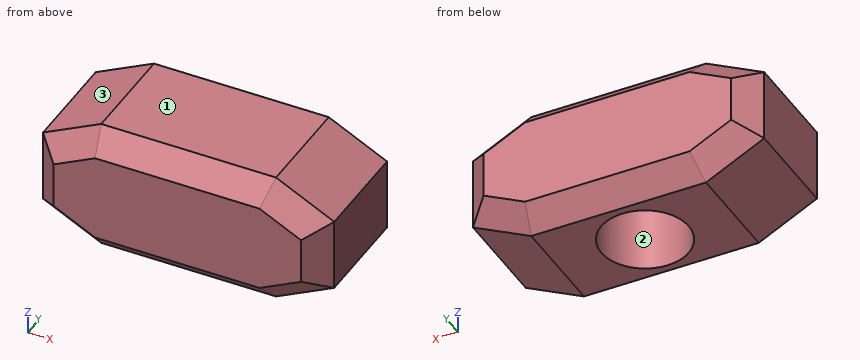
from build123d import *

# Parameters (mm, degrees)
F1_DEPTH = 20
F2_SIZE  = 3
F3_R     = 6
F4_DEPTH = 10
F5_R     = 0.5


with BuildPart() as f1:
    # F0 (on Front) → F1 (new body)
    with BuildSketch(Plane.XZ):
        Polygon((0, 4), (8, 0), (32, 0), (40, 4), (40, 14), (32, 18), (8, 18), (0, 14), align=None)
    extrude(amount=F1_DEPTH)

    # F2
    f2_edges = [f1.edges().sort_by_distance(p)[0] for p in [
        (4, -20, 2),
        (20, -20, 0),
        (36, -20, 2),
        (40, -20, 9),
        (36, -20, 16),
        (20, -20, 18),
        (4, -20, 16),
        (0, -20, 9),
        (4, 0, 2),
        (20, 0, 0),
        (36, 0, 2),
        (40, 0, 9),
        (36, 0, 16),
        (20, 0, 18),
        (4, 0, 16),
        (0, 0, 9),
    ]]
    chamfer(f2_edges, length=F2_SIZE)

    # F3 (on face) → F4 (cut)
    with BuildSketch(Plane(origin=(0, 0, 0), x_dir=(1, 0, 0), z_dir=(0, 0, -1))):
        with Locations((20, 10)):
            Circle(F3_R)
    extrude(amount=-F4_DEPTH, mode=Mode.SUBTRACT)

    # F5
    f5_edges = [f1.edges().sort_by_distance(p)[0] for p in [
        (14, -10, 10),
    ]]
    fillet(f5_edges, radius=F5_R)


solid = f1.part
Work out the finished part from the listing and answer in its coordinate system (mm). Face numbers are marked on the shaded views. Give positions to 0.01 mm unless a question says otherwise; leave off trailing zeros. Write each loop counter-clockwise with the first axis right and the second up, starting at its lowest first coordinate (ties: lowest second). Pieces come first, ordered by that corner, then holes. Notation, with made-up numbers: (35.5, 81.5) - (67.5, 81.5) arc R24 ccw to (67.5, 112.5) - close; hole circle Ø3 at (-23, 86.25). An arc over 180 degrees is marked (long way). One line per item, written item: value. Start each with the question number.
1. Find section D-D (x = 20). Write down the section's boundary in (y, z), then the cut area to 3 significant figures.
2. For a pull along X with two mould halves and no side action, classify the marked faces 1, 2 and 3 as +X half, -X half, draft (parallel to the pull), parting line (faces both ways), or undercut.
3. Given pin 1 (1.5 mm diameter, centred on y = -6.5, z = 15, fed in from -X); pin 2 (5.5 mm diameter, centred on x = 19.5, y = -11, fed in from -Z), each flat-ended and moving along its own axis, determine where each tip first touches the part or whether it passes through.
4. Find section B-B (x = 28). Write down the section's boundary in (y, z), then the cut area to 3 significant figures.
5. Consider probe 1 along X at (y, z) = (-10, 6.5); probe 2 along Y at (x, z) = (20, 3.25); probe 3 along X at (y, z) = (-8.25, 1.75). Determine where each line is inside the solid, lowest interval first.
6. Find section A-A (z = 6.5). Write down the section's boundary in (x, y).
7. Find section C-C (y = -10). Write down the section's boundary in (x, z), then the cut area to 3 significant figures.
Geometry results:
1. outline: (-20, 3) - (-17, 0) - (-16, 0) - (-16, 9.5) arc R0.5 cw to (-15.5, 10) - (-4.5, 10) arc R0.5 cw to (-4, 9.5) - (-4, 0) - (-3, 0) - (0, 3) - (0, 15) - (-3, 18) - (-17, 18) - (-20, 15) - close
1. area: 222 mm2
2. face 1: draft
2. face 2: undercut
2. face 3: -X half
3. pin 1: x = 0.5
3. pin 2: z = 10
4. outline: (-20, 3) - (-17, 0) - (-3, 0) - (0, 3) - (0, 15) - (-3, 18) - (-17, 18) - (-20, 15) - close
4. area: 342 mm2
5. probe 1: 0 to 14, 26 to 40
5. probe 2: -20 to -16, -4 to 0
5. probe 3: 4.5 to 14.26, 25.74 to 35.5
6. outline: (0, -17) - (3, -20) - (37, -20) - (40, -17) - (40, -3) - (37, 0) - (3, 0) - (0, -3) - close; hole circle Ø12 at (20, -10)
7. outline: (0, 4) - (8, 0) - (14, 0) - (14, 9.5) arc R0.5 cw to (14.5, 10) - (25.5, 10) arc R0.5 cw to (26, 9.5) - (26, 0) - (32, 0) - (40, 4) - (40, 14) - (32, 18) - (8, 18) - (0, 14) - close
7. area: 536 mm2
